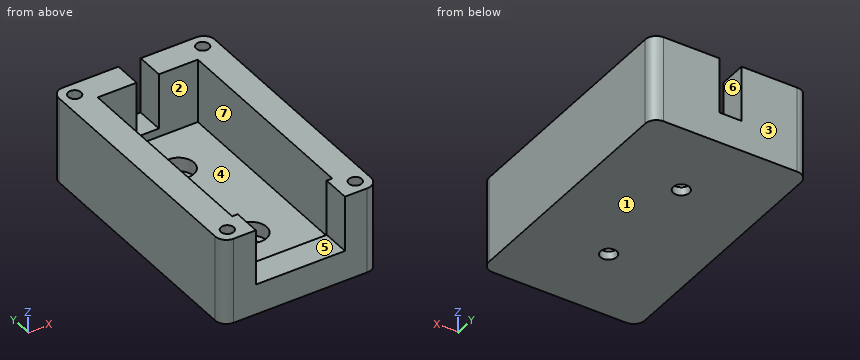
from build123d import *

# Parameters (mm, degrees)
F0_W           = 28
F0_H           = 47
F0_R           = 1.15
F0_W_2         = 18
F0_H_2         = 37
F1_DEPTH       = 11.5
F2_W           = 28
F2_H           = 47
F2_R           = 1.15
F2_W_2         = 18
F2_H_2         = 37
F3_DEPTH       = 4
F4_W           = 16
F4_H           = 5
F4_W_2         = 4
F5_DEPTH       = 10
F6_R           = 2
F8_D           = 2.9
F8_CBORE_D     = 5.5
F8_CBORE_DEPTH = 2.5


with BuildPart() as f1:
    # F0 (on Top) → F1 (new body)
    with BuildSketch(Plane.XY):
        Rectangle(F0_W, F0_H)
        with Locations((-11.5, -21)):
            Circle(F0_R, mode=Mode.SUBTRACT)
        with Locations((11.5, -21)):
            Circle(F0_R, mode=Mode.SUBTRACT)
        with Locations((-11.5, 21)):
            Circle(F0_R, mode=Mode.SUBTRACT)
        Rectangle(F0_W_2, F0_H_2, mode=Mode.SUBTRACT)
        with Locations((11.5, 21)):
            Circle(F0_R, mode=Mode.SUBTRACT)
    extrude(amount=F1_DEPTH)

    # F2 (on face) → F3 (join)
    with BuildSketch(Plane(origin=(0, 0, 0), x_dir=(1, 0, 0), z_dir=(0, 0, -1))):
        Rectangle(F2_W, F2_H)
        with Locations((-11.5, -21)):
            Circle(F2_R, mode=Mode.SUBTRACT)
        with Locations((11.5, -21)):
            Circle(F2_R, mode=Mode.SUBTRACT)
        with Locations((-11.5, 21)):
            Circle(F2_R, mode=Mode.SUBTRACT)
        Rectangle(F2_W_2, F2_H_2, mode=Mode.SUBTRACT)
        with Locations((11.5, 21)):
            Circle(F2_R, mode=Mode.SUBTRACT)
        with Locations((-11.5, 21)):
            Circle(F2_R)
        with Locations((11.5, 21)):
            Circle(F2_R)
        with Locations((-11.5, -21)):
            Circle(F2_R)
        Rectangle(F2_W_2, F2_H_2)
        with Locations((11.5, -21)):
            Circle(F2_R)
    extrude(amount=F3_DEPTH)

    # F4 (on face) → F5 (cut)
    with BuildSketch(Plane.XY.offset(11.5)):
        with Locations((0, -21)):
            Rectangle(F4_W, F4_H)
        with Locations((0, 21)):
            Rectangle(F4_W_2, F4_H)
    extrude(amount=-F5_DEPTH, mode=Mode.SUBTRACT)

    # F6
    f6_edges = [f1.edges().sort_by_distance(p)[0] for p in [
        (-14, 23.5, 3.75),
        (14, 23.5, 3.75),
        (14, -23.5, 3.75),
        (-14, -23.5, 3.75),
    ]]
    fillet(f6_edges, radius=F6_R)

    # F8 (through all)
    with Locations(Plane.XY):
        with Locations((0, 10), (0, -10)):
            CounterBoreHole(F8_D / 2, F8_CBORE_D / 2, F8_CBORE_DEPTH)


solid = f1.part
The listing builds one solid part. Answer for the finished solid, in the listing's coordinates (mm). Face numbers are marked on the shaded views. A direction names the side the tool comes from. Coordinates: 2 decimals unless noted, no trailing zeros. Loops run counter-clockwise (first coordinate to the right, second up) from the corner with the lowest first, then second, coordinate; pieces in that order, holes last.
1) Find section A-A on z = 7. Write down the section's boundary in (x, y).
2) Find section B-B on x = 0. Write down the section's boundary in (y, z), then the cut area to 3 significant figures.
3) Find section D-D on y = -21. Write down the section's boundary in (x, z).
4) Determine the mould class of the marked faces 1, 2, 3 and 4 for opening direction Y: pulls with the +Y half, pulls with the -Y half, needs draft (parallel to the pull), parting line crosses it, or undercut.
5) Find section C-C on y = -10. Write down the section's boundary in (x, z).
6) Flat-ended cylindrical pins translate along their axes: pin 1 Ø9 at (x, y) = (-3, 9) entering from +Z; pin 2 Ø2 at (x, z) = (3.5, 8.5) entering from -Y; pin 3 Ø4.5 at (x, y) = (0, -10) entering from +Z; pin 4 Ø2.5 at (x, y) = (0, 10) entering from -Z. Find the tip coordinate at first contact, or state that the pin passes through.
7) Find the intervals of material crossed by L1, parallel to Y at x = 0, z = -0.7; L2, parallel to Y at x = -11.5, z = 5.5; L3, parallel to X at y = 10.5, z = 9.5, in increasing order.
8) A tool of negligible diameter and unlimited length cuts with its end or side. For the marked faces 5, 6 and 7, from which of +Z, -Z, +X, -X, +Y, -Y can it reach the whole face along a straight path? Write none if from no direction.
Values:
1. outline: (-14, -21.5) arc R2 ccw to (-12, -23.5) - (-8, -23.5) - (-8, -18.5) - (-9, -18.5) - (-9, 18.5) - (-2, 18.5) - (-2, 23.5) - (-12, 23.5) arc R2 ccw to (-14, 21.5) - close; (2, 18.5) - (9, 18.5) - (9, -18.5) - (8, -18.5) - (8, -23.5) - (12, -23.5) arc R2 ccw to (14, -21.5) - (14, 21.5) arc R2 ccw to (12, 23.5) - (2, 23.5) - close; hole circle Ø2.3 at (-11.5, -21); hole circle Ø2.3 at (-11.5, 21); hole circle Ø2.3 at (11.5, -21); hole circle Ø2.3 at (11.5, 21)
2. outline: (-23.5, -4) - (-11.45, -4) - (-11.45, -2.5) - (-12.75, -2.5) - (-12.75, 0) - (-18.5, 0) - (-18.5, 1.5) - (-23.5, 1.5) - close; (-8.55, -4) - (8.55, -4) - (8.55, -2.5) - (7.25, -2.5) - (7.25, 0) - (-7.25, 0) - (-7.25, -2.5) - (-8.55, -2.5) - close; (11.45, -4) - (23.5, -4) - (23.5, 1.5) - (18.5, 1.5) - (18.5, 0) - (12.75, 0) - (12.75, -2.5) - (11.45, -2.5) - close
2. area: 167 mm2
3. outline: (-14, -4) - (14, -4) - (14, 11.5) - (12.65, 11.5) - (12.65, 0) - (10.35, 0) - (10.35, 11.5) - (8, 11.5) - (8, 1.5) - (-8, 1.5) - (-8, 11.5) - (-10.35, 11.5) - (-10.35, 0) - (-12.65, 0) - (-12.65, 11.5) - (-14, 11.5) - close
4. face 1: needs draft
4. face 2: undercut
4. face 3: pulls with the +Y half
4. face 4: undercut
5. outline: (-14, -4) - (-1.45, -4) - (-1.45, -2.5) - (-2.75, -2.5) - (-2.75, 0) - (-9, 0) - (-9, 11.5) - (-14, 11.5) - close; (1.45, -4) - (14, -4) - (14, 11.5) - (9, 11.5) - (9, 0) - (2.75, 0) - (2.75, -2.5) - (1.45, -2.5) - close
6. pin 1: stops at z = 0
6. pin 2: stops at y = 18.5
6. pin 3: stops at z = -2.5
6. pin 4: passes through
7. L1: y = -23.5 to -12.75, -7.25 to 7.25, 12.75 to 23.5
7. L2: y = -23.5 to -22.15, -19.85 to 19.85, 22.15 to 23.5
7. L3: x = -14 to -9, 9 to 14
8. face 5: +Z, -Y
8. face 6: +Z, +Y, -Y
8. face 7: +Z
